Could you check a few things on this model? Use its own coordinates, in mm. Face numbers are marked on the shaded views. Give positions to 0.01 mm unless a question says otherwise; leave off trailing zeros. Loops run counter-clockwise (first coordinate to the right, second up) from the corner with the lowest first, then second, coordinate; pieces in that order, holes last. Notation, with made-up numbers: (-37, 88) - (4, 88) arc R17 cw to (4, 120) - close; hole circle Ø2 at (-4, -8). An arc over 180 degrees is marked (long way). One line per item, written item: value. Start each with the question number.
Q1. If we mould it in two halves opening along Z, with no side actions, what happens to the marked faces 1 and 2? For each: released by +Z, released by -Z, zero draft, split by the parting line, or undercut.
Q2. I want a section at A-A (z = 0). Please give me the cut outline in (x, y).
Q3. I want a section at C-C (z = -83.5). Please give me the cut outline in (x, y).
Q4. I want a section at B-B (x = 0). Count the separate pieces of the cut face and the enclosed holes in it, then the cut area to 3 significant figures.
Q5. If I drill on line 1 (X direction, y = -0.5, z = -93); line 2 (Y direction, x = -8, z = -175); line 3 (Z direction, x = 8, y = 0.5), over which ranges is the centre line in solid material (lowest first)? Write a range as from..to.
Q6. I'm going to push flat-ended pins straight in: P1, Ø16, axis at x = 0, z = -18, coming from the +Y side; P2, Ø3, axis at x = 10, y = 4, coming from the +Z side; P3, Ø7, axis at x = 0, z = -18, coming from the +Y side; P4, Ø12, axis at x = 4, y = -6, coming from the +Z side. Where does each tip first touch, or does it pass through?
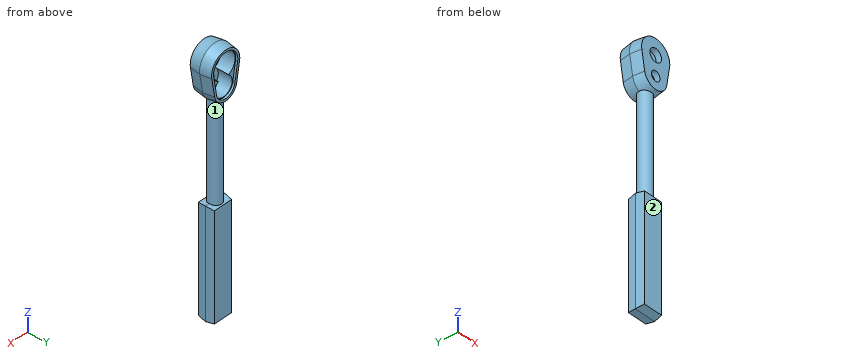
```python
from build123d import *

# Parameters (mm, degrees)
CROQUIS1_W                        = 20
CROQUIS1_H                        = 100
MANGO_DEPTH                       = 7.5
MANGO_TAPER                       = 8
MANGO_OTHER_WAY_DEPTH             = 7.5
MANGO_OTHER_WAY_TAPER             = 8
TRANSICION_REACH                  = 222.355
CROQUIS2_R                        = 6
SALIENTE_EXTRUIR3_DEPTH           = 10
SALIENTE_EXTRUIR3_TAPER           = 8
SALIENTE_EXTRUIR3_OTHER_WAY_DEPTH = 10
SALIENTE_EXTRUIR3_OTHER_WAY_TAPER = 8
CORTAR_EXTRUIR1_DEPTH             = 2
CORTAR_EXTRUIR2_DEPTH             = 13
CROQUIS6_R                        = 4.5
CORTAR_EXTRUIR3_DEPTH             = 5
CROQUIS7_R                        = 6
CORTAR_EXTRUIR4_DEPTH             = 5


with BuildPart() as part:
    # Croquis1 → Mango (new body)
    with BuildSketch(Plane(origin=(0, 0, 0), x_dir=(1, 0, 0), z_dir=(0, 1, 0))):
        with Locations((0, 170)):
            Rectangle(CROQUIS1_W, CROQUIS1_H)
    extrude(amount=MANGO_DEPTH, taper=MANGO_TAPER)

    # Croquis1 → Mango other way (add)
    with BuildSketch(Plane(origin=(0, 0, 0), x_dir=(1, 0, 0), z_dir=(0, 1, 0))):
        with Locations((0, 170)):
            Rectangle(CROQUIS1_W, CROQUIS1_H)
    extrude(amount=-MANGO_OTHER_WAY_DEPTH, taper=MANGO_OTHER_WAY_TAPER)

    # Croquis2 → Transicion (add, up to next)
    with BuildSketch(Plane.XY, mode=Mode.PRIVATE) as transicion_sk1:
        Circle(CROQUIS2_R)
    transicion_tool1 = extrude(transicion_sk1.sketch, amount=-TRANSICION_REACH, mode=Mode.PRIVATE) - part.part
    add(transicion_tool1.solids().sort_by_distance((0, 0, 0))[0])

    # Croquis3 → Saliente-Extruir3 (add)
    with BuildSketch(Plane(origin=(0, 0, 0), x_dir=(1, 0, 0), z_dir=(0, 1, 0))):
        with BuildLine():
            ThreePointArc((12.818172863, 20.166666667), (0, 31), (-12.818172863, 20.166666667))
            Line((-12.818172863, 20.166666667), (-15.776212755, 2.666666667))
            ThreePointArc((-15.776212755, 2.666666667), (0, -16), (15.776212755, 2.666666667))
            Line((15.776212755, 2.666666667), (12.818172863, 20.166666667))
        make_face()
    extrude(amount=SALIENTE_EXTRUIR3_DEPTH, taper=SALIENTE_EXTRUIR3_TAPER)

    # Croquis3 → Saliente-Extruir3 other way (add)
    with BuildSketch(Plane(origin=(0, 0, 0), x_dir=(1, 0, 0), z_dir=(0, 1, 0))):
        with BuildLine():
            ThreePointArc((12.818172863, 20.166666667), (0, 31), (-12.818172863, 20.166666667))
            Line((-12.818172863, 20.166666667), (-15.776212755, 2.666666667))
            ThreePointArc((-15.776212755, 2.666666667), (0, -16), (15.776212755, 2.666666667))
            Line((15.776212755, 2.666666667), (12.818172863, 20.166666667))
        make_face()
    extrude(amount=-SALIENTE_EXTRUIR3_OTHER_WAY_DEPTH, taper=SALIENTE_EXTRUIR3_OTHER_WAY_TAPER)

    # Croquis4 → Cortar-Extruir1 (cut)
    with BuildSketch(Plane(origin=(0, 10, 0), x_dir=(1, 0, 0), z_dir=(0, 1, 0))):
        with BuildLine():
            Line((-9.460394951, 19.599098609), (-12.418434842, 2.099098609))
            ThreePointArc((-12.418434842, 2.099098609), (0, -12.594591653), (12.418434842, 2.099098609))
            Line((12.418434842, 2.099098609), (9.460394951, 19.599098609))
            ThreePointArc((9.460394951, 19.599098609), (0, 27.594591653), (-9.460394951, 19.599098609))
        make_face()
    extrude(amount=-CORTAR_EXTRUIR1_DEPTH, mode=Mode.SUBTRACT)

    # Croquis5 → Cortar-Extruir2 (cut)
    with BuildSketch(Plane(origin=(0, 8, 0), x_dir=(1, 0, 0), z_dir=(0, 1, 0))):
        with BuildLine():
            ThreePointArc((5.332682252, 10.75), (0, 27), (-5.332682252, 10.75))
            ThreePointArc((-5.332682252, 10.75), (0, -12), (5.332682252, 10.75))
        make_face()
    extrude(amount=-CORTAR_EXTRUIR2_DEPTH, mode=Mode.SUBTRACT)

    # Croquis6 → Cortar-Extruir3 (cut)
    with BuildSketch(Plane(origin=(0, -5, 0), x_dir=(1, 0, 0), z_dir=(0, 1, 0))):
        with Locations(Location((0, 18, 0), (0, 0, 270))):
            Circle(CROQUIS6_R)
    extrude(amount=-CORTAR_EXTRUIR3_DEPTH, mode=Mode.SUBTRACT)

    # Croquis7 → Cortar-Extruir4 (cut)
    with BuildSketch(Plane(origin=(0, -5, 0), x_dir=(1, 0, 0), z_dir=(0, 1, 0))):
        with Locations(Location((0, 0, 0), (0, 0, 270))):
            Circle(CROQUIS7_R)
    extrude(amount=-CORTAR_EXTRUIR4_DEPTH, mode=Mode.SUBTRACT)


solid = part.part
```
Worked answers:
1. face 1: undercut
1. face 2: zero draft
2. outline: (-16, 0) - (-14.59, -10) - (-6, -10) - (-6, -5) - (-12, -5) - (-12, 8) - (-12.59, 8) - (-12.59, 10) - (-14.59, 10) - close; (6, -10) - (14.59, -10) - (16, 0) - (14.59, 10) - (12.59, 10) - (12.59, 8) - (12, 8) - (12, -5) - (6, -5) - close
3. outline: circle Ø12 at (0, 0)
4. separate pieces: 3
4. enclosed holes: 0
4. area: 2,780 mm²
5. line 1: x = -5.98..5.98
5. line 2: y = -7.5..7.5
5. line 3: z = -219.93..-120.07, -28.16..-22.12, -13.88..-8.94, 8.94..13.78
6. P1: stops at y = -5
6. P2: stops at z = 12.92
6. P3: passes through
6. P4: stops at z = 15.86
